Could you check a few things on this model? Use its own coordinates, in mm. A direction names the side the tool comes from. Coordinates: 2 decimals unless noted, no trailing zeros. Loops run counter-clockwise (first coordinate to the right, second up) from the corner with the lowest first, then second, coordinate; pieces in that order, holes last. Notation, with made-up numbers: (38, -29.75) -> (63, -29.75) arc R19 ccw to (63, 4.25) -> close; hole circle Ø4 at (-20, 78). An arc over 180 degrees is marked (long way). One line per question, with ' | ' between items.
from build123d import *

# Parameters (mm, degrees)
SKETCH1_W           = 300
SKETCH1_H           = 200
BOSS_EXTRUDE1_DEPTH = 200
SKETCH2_R           = 14
BOSS_EXTRUDE2_DEPTH = 25
SKETCH3_R           = 60
BOSS_EXTRUDE3_DEPTH = 5
SKETCH4_R           = 14
BOSS_EXTRUDE4_DEPTH = 15
FILLET1_R           = 5
SKETCH5_W           = 200
SKETCH5_H           = 200
BOSS_EXTRUDE5_DEPTH = 5
SKETCH6_R           = 57
BOSS_EXTRUDE6_DEPTH = 2300


with BuildPart() as part:
    # Sketch1 → Boss-Extrude1 (new body)
    with BuildSketch(Plane(origin=(0, 0, 0), x_dir=(1, 0, 0), z_dir=(0, 1, 0))):
        Rectangle(SKETCH1_W, SKETCH1_H)
    extrude(amount=BOSS_EXTRUDE1_DEPTH)

    # Sketch2 → Boss-Extrude2 (add)
    with BuildSketch(Plane(origin=(150, 0, 0), x_dir=(0, 0, -1), z_dir=(1, 0, 0))):
        with Locations((0, 100)):
            Circle(SKETCH2_R)
    extrude(amount=BOSS_EXTRUDE2_DEPTH)

    # Sketch3 → Boss-Extrude3 (add)
    with BuildSketch(Plane(origin=(175, 0, 0), x_dir=(0, 0, -1), z_dir=(1, 0, 0))):
        with Locations((0, 100)):
            Circle(SKETCH3_R)
    extrude(amount=BOSS_EXTRUDE3_DEPTH)

    # Sketch4 → Boss-Extrude4 (add)
    with BuildSketch(Plane(origin=(180, 0, 0), x_dir=(0, 0, -1), z_dir=(1, 0, 0))):
        with Locations((0, 100)):
            Circle(SKETCH4_R)
    extrude(amount=BOSS_EXTRUDE4_DEPTH)

    # Fillet1
    fillet1_edges = [part.edges().sort_by_distance(p)[0] for p in [
        (195, 100, 14),
    ]]
    fillet(fillet1_edges, radius=FILLET1_R)

    # Sketch5 → Boss-Extrude5 (add)
    with BuildSketch(Plane.XZ):
        Rectangle(SKETCH5_W, SKETCH5_H)
    extrude(amount=BOSS_EXTRUDE5_DEPTH)

    # Sketch6 → Boss-Extrude6 (add)
    with BuildSketch(Plane.XZ.offset(5)):
        Circle(SKETCH6_R)
    extrude(amount=BOSS_EXTRUDE6_DEPTH)


solid = part.part
1) We'd pull the mould along X, two halves only. Please class faces 1 (the face through (150, 76, 1)), 2 (the face through (-150, 99, 1)), 3 (the face through (175, 114.2, 0.8)), 4 (the face through (125, 0, -1)): pulls with the +X half, pulls with the -X half, needs draft (parallel to the pull), parting line crosses it, or undercut.
Data:
face 1: undercut | face 2: pulls with the -X half | face 3: undercut | face 4: needs draft
2) On a 3-axis mill with a long thin cutter (end or side, diameter ignored), from which of +Z, -Z, +X, -X, +Y, -Y can I reach the whole of each face in a straight line? I mean faces 5 (the face through (177.465, 41.427, 13.007)), 6 (the face through (-46, -5, 46)), 7 (the face through (-125, 0, -1)). Say none if no direction works.
Data:
face 5: +X | face 6: -Y | face 7: +Z, -Z, -X, -Y
3) I'm going to push flat-ended pins straight in: pin 1 Ø12 at (x, y) = (-10, -1806) entering from -Z; pin 2 Ø10 at (y, z) = (-869, -7.5) entering from -X; pin 3 Ø1.5 at (y, z) = (-3.5, -21) entering from -X. Where does each tip first touch, or does it pass through?
Data:
pin 1: z = -56.86 | pin 2: x = -56.95 | pin 3: x = -100
4) If we section it at B-B on y = -1058.5: Please give me the cut outline in (x, z).
Data:
outline: circle Ø114 at (0, 0)
5) I need wall thicknesses on line 1 along Y through (x, z) = (-102, -60); line 2 along Y through (x, z) = (-94, -61); line 3 along X through (y, z) = (-657.5, 22). Which ranges of each line are inside material? Lowest first, please. Write a range as from..to.
Data:
line 1: 0..200 | line 2: -5..200 | line 3: -52.58..52.58
6) If we section it at A-A on x = 0: Please give me the cut outline in (y, z).
Data:
outline: (-2305, -57) -> (-5, -57) -> (-5, -100) -> (200, -100) -> (200, 100) -> (-5, 100) -> (-5, 57) -> (-2305, 57) -> close
